from build123d import *

# Parameters (mm, degrees)
CROQUIS1_R              = 3.0226
SALIENTE_EXTRUIR1_DEPTH = 5.334


with BuildPart() as part:
    # Croquis1 → Saliente-Extruir1 (new body)
    with BuildSketch(Plane(origin=(0, 0, 0), x_dir=(1, 0, 0), z_dir=(0, 1, 0))):
        Polygon((-6.26182555, 0), (-3.130912775, -5.4229), (3.130912775, -5.4229), (6.26182555, 0), (3.130912775, 5.4229), (-3.130912775, 5.4229), align=None)
        with Locations(Location((0, 0, 0), (0, 0, 270))):
            Circle(CROQUIS1_R, mode=Mode.SUBTRACT)
    extrude(amount=SALIENTE_EXTRUIR1_DEPTH)

    # Croquis2 → Cortar-Revolución1 (revolve, cut)
    with BuildSketch(Plane.XY, mode=Mode.PRIVATE) as cortar_revoluci_n1_sk:
        Polygon((-6.26182555, 5.334), (-6.26182555, 4.834), (-5.26182555, 5.334), align=None)
    revolve(cortar_revoluci_n1_sk.sketch.rotate(Axis((0, 0, 0), (0, 1, 0)), 270), axis=Axis((0, 0, 0), (0, 1, 0)), mode=Mode.SUBTRACT)

    # Croquis3 → Cortar-Revolución3 (revolve, cut)
    with BuildSketch(Plane.XY, mode=Mode.PRIVATE) as cortar_revoluci_n3_sk:
        Polygon((-6.26182555, 0), (-5.26182555, 0), (-6.26182555, 0.5), align=None)
    revolve(cortar_revoluci_n3_sk.sketch.rotate(Axis((0, 0, 0), (0, 1, 0)), 120.000000008), axis=Axis((0, 0, 0), (0, 1, 0)), mode=Mode.SUBTRACT)


solid = part.part
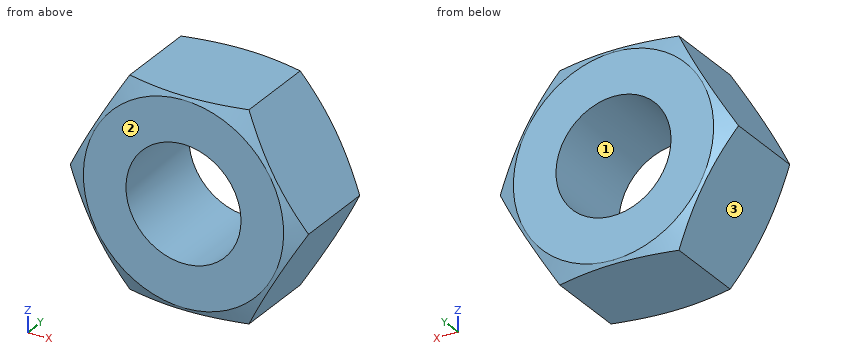
Can you work these out from the model? Positions are in its coordinate system, mm. Face numbers are marked on the shaded views. Round coordinates to 2 decimals unless told otherwise and drop trailing zeros. Loops run counter-clockwise (first coordinate to the right, second up) from the corner with the lowest first, then second, coordinate; pieces in that order, holes last. Notation, with made-up numbers: (39.5, 11.5) - (76.5, 11.5) arc R23 cw to (76.5, 49.5) - close; hole circle Ø6 at (-13, -2.75). An arc over 180 degrees is marked (long way). Answer in a Markdown table with one row per item. Add a question column.
Q1. I need wall thicknesses on L1, parallel to Z at x = 2, y = 0.5; L2, parallel to Z at x = -2.5, y = 1.2; L3, parallel to X at y = 3.95, z = 1.5. Which ranges of each line are inside material? Lowest first, please.
Q2. For pin 1 Ø3 at (y, z) = (3, -3.5) entering from +X; pin 2 Ø1 at (y, z) = (4.5, 1.5) entering from +X, each with a flat end and sliding along its axis, tell me the tip position at first contact or that it passes through.
Q3. We'd pull the mould along Z, two halves only. Please class the marked faces 1, 2 and 3: pulls with the +Z half, pulls with the -Z half, needs draft (parallel to the pull), parting line crosses it, or undercut.
Q4. I want a section at A-A on y = 2.25. List the corners of the cut face in (x, z) for me, and give its area (3 significant figures).
Q5. I want a section at B-B on x = 0. List the corners of the cut face in (y, z) for me.
A:
| question | item | result |
|---|---|---|
| 1 | L1 | -5.42 to -2.27, 2.27 to 5.42 |
| 1 | L2 | -5.42 to -1.7, 1.7 to 5.42 |
| 1 | L3 | -5.4 to -2.62, 2.62 to 5.4 |
| 2 | pin 1 | x = 5.11 |
| 2 | pin 2 | x = 5.68 |
| 3 | face 1 | undercut |
| 3 | face 2 | needs draft |
| 3 | face 3 | pulls with the -Z half |
| 4 | outline | (-6.26, 0) - (-3.13, -5.42) - (3.13, -5.42) - (6.26, 0) - (3.13, 5.42) - (-3.13, 5.42) - close; hole circle Ø6.05 at (0, 0) |
| 4 | area | 73.2 mm^2 |
| 5 | outline | (0, -5.26) - (0.08, -5.42) - (5.25, -5.42) - (5.33, -5.26) - (5.33, -3.02) - (0, -3.02) - close; (0, 3.02) - (5.33, 3.02) - (5.33, 5.26) - (5.25, 5.42) - (0.08, 5.42) - (0, 5.26) - close |
